```python
from build123d import *

# Parameters (mm, degrees)
F0_W     = 203.2
F0_H     = 127
F1_DEPTH = 127
F3_DEPTH = 76.2
F4_SIZE2 = 101.6
F4_SIZE  = 76.2
F5_R     = 5.08


with BuildPart() as f1:
    # F0 (on Front) → F1 (new body)
    with BuildSketch(Plane.XZ):
        with Locations((8.8248885557, -5.8830874041)):
            Rectangle(F0_W, F0_H)
    extrude(amount=F1_DEPTH)

    # F2 (on face) → F3 (cut)
    with BuildSketch(Plane.XZ.offset(127)):
        Polygon((110.4248885557, 57.6169125959), (8.8248885557, 57.6169125959), (8.8248885557, -3.765176516), (-29.2751114443, -3.765176516), (-29.2751114443, -69.3830874041), (110.4248885557, -69.3830874041), align=None)
    extrude(amount=-F3_DEPTH, mode=Mode.SUBTRACT)

    # F4
    f4_edges = [f1.edges().sort_by_distance(p)[0] for p in [
        (110.424889, -25.4, 57.616913),
    ]]
    f4_side = f1.faces().sort_by_distance((-12.94654, -52.614286, 57.616913))[0]
    chamfer(f4_edges, length=F4_SIZE, length2=F4_SIZE2, reference=f4_side)

    # F5
    f5_edges = [f1.edges().sort_by_distance(p)[0] for p in [
        (-41.975111, -127, 57.616913),
        (8.824889, -88.9, 57.616913),
        (21.524889, -50.8, 57.616913),
        (34.224889, -25.4, 57.616913),
        (8.824889, -50.8, 26.925868),
        (8.824889, -127, 26.925868),
        (-10.225111, -127, -3.765177),
        (8.824889, -88.9, -3.765177),
        (-29.275111, -127, -36.574132),
        (-29.275111, -50.8, -36.574132),
        (-61.025111, -127, -69.383087),
        (-29.275111, -88.9, -69.383087),
        (40.574889, -50.8, -69.383087),
        (110.424889, -25.4, -69.383087),
        (-92.775111, -127, -5.883087),
        (8.824889, 0, -69.383087),
        (-92.775111, 0, -5.883087),
        (-10.225111, -50.8, -3.765177),
    ]]
    fillet(f5_edges, radius=F5_R)


solid = f1.part
```
For this review, take the finished solid that the model builds, in its own axes (mm). A direction names the side the tool comes from. Coordinates: 2 decimals unless noted, no trailing zeros. Order: outer loops, then holes, each group sorted by start corner. A loop starts at its lowest first (then second) coordinate and runs counter-clockwise, first axis right, second up. Notation, with made-up numbers: (-39, 6) -> (-28, 6) arc R20 cw to (-28, 41) -> close; hole circle Ø9 at (54, -24.75). An arc over 180 degrees is marked (long way). Answer as CSV lines item,"result".
Q1. We need section A-A (y = -119). State the section outline as (x, z) points, plus the area to 3 significant figures.
Model answer:
outline,"(-92.78, -69.38) -> (-34.36, -69.38) arc R5.08 ccw to (-29.28, -64.3) -> (-29.28, -3.77) -> (3.74, -3.77) arc R5.08 ccw to (8.82, 1.31) -> (8.82, 52.54) arc R5.08 ccw to (3.74, 57.62) -> (-92.78, 57.62) -> close"
area,"10,400 mm2"
Q2. Draft analysis for pull direction Y (two halves, no side actions). For faces 4 (the face through (-12, 0, -2)), 5 (the face through (7.376, -88.438, -2.238)), 6 (the face through (-63.156, -125.551, -67.855)), state which applies: released by +Y, released by -Y, zero draft, split by the parting line, or undercut.
Model answer:
face 4,"released by +Y"
face 5,"zero draft"
face 6,"released by -Y"
Q3. Clearance check with flat-ended pins moving along their axes: pin 1 Ø15.5 at (y, z) = (-100.5, 27) entering from +X; pin 2 Ø2 at (y, z) = (-89.5, -12.5) entering from +X. State where each tip first meets the part, or that it passes through.
Model answer:
pin 1,"stops at x = 8.82"
pin 2,"stops at x = -29.28"
Q4. We need section C-C (y = -14). State the section outline as (x, z) points, plus the area to 3 significant figures.
Model answer:
outline,"(-92.78, -69.38) -> (105.34, -69.38) arc R5.08 ccw to (110.42, -64.3) -> (110.42, -43.98) -> (35.75, 55.58) arc R5.08 ccw to (31.68, 57.62) -> (-92.78, 57.62) -> close"
area,"21,900 mm2"
Q5. We need section B-B (z = -49.5). State the section outline as (x, y) points.
Model answer:
outline,"(-92.78, -121.92) arc R5.08 ccw to (-87.7, -127) -> (-34.36, -127) arc R5.08 ccw to (-29.28, -121.92) -> (-29.28, -55.88) arc R5.08 cw to (-24.2, -50.8) -> (110.42, -50.8) -> (110.42, 0) -> (-87.7, 0) arc R5.08 ccw to (-92.78, -5.08) -> close"
Q6. Wall thickness on line 1 along Y through (x, z) = (65.5, -50.5); line 2 along Z through (x, y) = (-6.5, -79); line 3 along X through (y, z) = (-96, -39): over which ranges is each line inside the solid? List them lowest first. Write a range as [from, to].
Model answer:
line 1,"y = [-50.8, 0]"
line 2,"z = [-3.77, 57.62]"
line 3,"x = [-92.78, -29.28]"
Q7. For faces 1 (the face through (-30.8, -125.55, -31.95)), 2 (the face through (10.4, -52.2, 26.6)), 3 (the face through (23.12, -49.27, 56.17)), list the 3-axis set-ups (+Z, -Z, +X, -X, +Y, -Y) from which the entire face can be reached by the end or side of a thin tool; tool diameter is ignored.
Model answer:
face 1,"-Z, +X, -Y"
face 2,"+Z, -Z, +X, -Y"
face 3,"+Z, +X, -Y"
Q8. We need section D-D (x = 58). State the section outline as (y, z) points, plus the area to 3 significant figures.
Model answer:
outline,"(-50.8, -64.3) arc R5.08 ccw to (-45.72, -69.38) -> (-5.08, -69.38) arc R5.08 ccw to (0, -64.3) -> (0, 25.92) -> (-50.8, 25.92) -> close"
area,"4,830 mm2"
